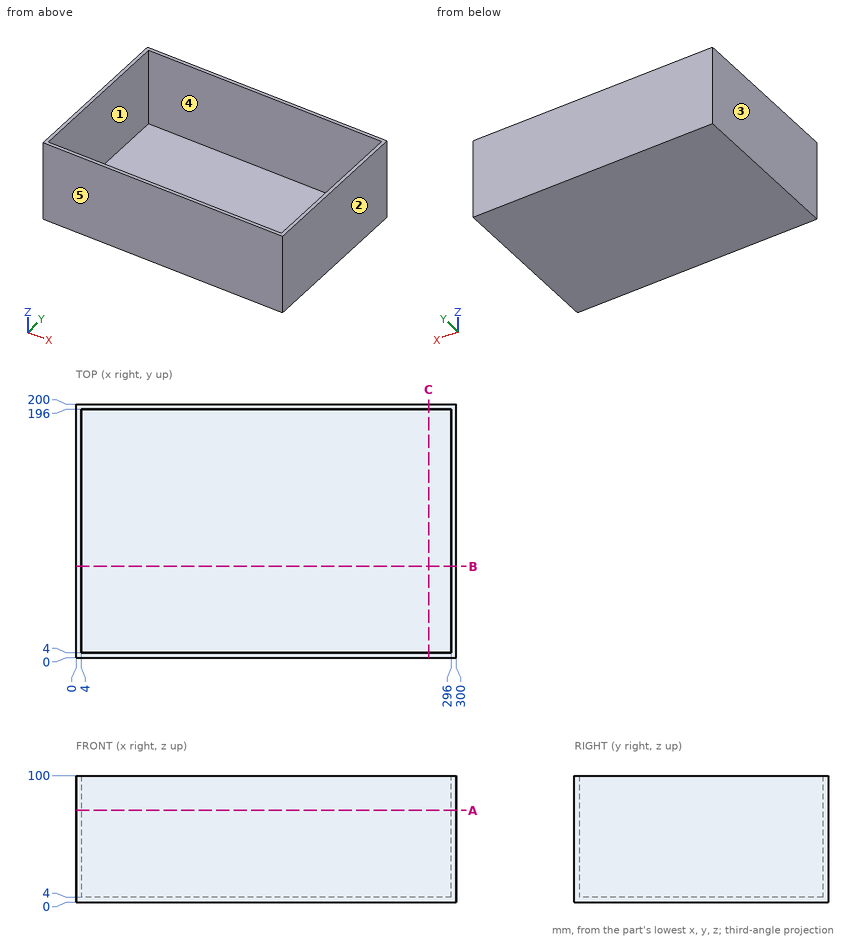
Design review of the part shown in the three views and the two pictorial views. Dimensions are in mm from the part's minimum x, y and z. A direction names the side the tool comes from. Round coordinates to 2 decimals unless told otherwise and drop trailing zeros. Loops run counter-clockwise (first coordinate to the right, second up) from the corner with the lowest first, then second, coordinate; pieces in that order, holes last.
Q1. To check wall thickness, follow line 1 along X through (y, z) = (171, 54); line 2 along Y through (x, z) = (88, 58); line 3 along Z through (x, y) = (42.5, 45.5). State the ranges of each line that lie inside material, in increasing order.
Result sheet:
line 1: x = 0 to 4, 296 to 300
line 2: y = 0 to 4, 196 to 200
line 3: z = 0 to 4
Q2. Machinability: for the marked faces 4 and 5, which of the approach directions +Z, -Z, +X, -X, +Y, -Y give a long, thin tool a straight path to every point of the face, cutting with its end or side? Answer none if there is none.
Result sheet:
face 4: +Z
face 5: +Z, -Z, +X, -X, -Y
Q3. Add section B-B on y = 72. Write out the cut boundary in (x, z), plus the area to 3 significant figures.
Result sheet:
outline: (0, 0) - (300, 0) - (300, 100) - (296, 100) - (296, 4) - (4, 4) - (4, 100) - (0, 100) - close
area: 1,970 mm2
Q4. Insertion check: pin 1 Ø5 at (x, y) = (143.5, 113) entering from +Z. The pin has a flat end and moves straight along its axis. Give the tip position at first contact, or say it passes through.
Result sheet:
pin 1: stops at z = 4
Q5. Mouldability with a two-part tool opening along X and no side actions: class the marked faces 1, 2 and 3 as +X half, -X half, draft (parallel to the pull), parting line (faces both ways), or undercut.
Result sheet:
face 1: undercut
face 2: +X half
face 3: -X half
Q6. Add section C-C on x = 278. Write out the cut boundary in (y, z).
Result sheet:
outline: (0, 0) - (200, 0) - (200, 100) - (196, 100) - (196, 4) - (4, 4) - (4, 100) - (0, 100) - close
Q7. Add section A-A on z = 72.5. Write out the cut boundary in (x, y), plus the area to 3 significant figures.
Result sheet:
outline: (0, 0) - (300, 0) - (300, 200) - (0, 200) - close; hole (4, 4) - (296, 4) - (296, 196) - (4, 196) - close
area: 3,940 mm2
